from build123d import *

# Parameters (mm, degrees)
SKETCH_1_R          = 50
SKETCH_1_R_2        = 45
EXTRUDE_1_DEPTH     = 12
FILLET_1_R          = 80
CUT_EXTRUDE_1_DEPTH = 12
SKETCH_4_W          = 6
SKETCH_4_H          = 50
CUT_EXTRUDE_2_DEPTH = 12


with BuildPart() as part:
    # 草图1 → 凸台-拉伸1 (new body)
    with BuildSketch(Plane(origin=(0, 0, 0), x_dir=(0, 0, -1), z_dir=(1, 0, 0))):
        with BuildLine():
            Line((-150, 75), (560.88072706, 75))
            Line((560.88072706, 75), (948, -121.211138337))
            Line((948, -121.211138337), (1008, -163))
            Line((1008, -163), (1008, -168))
            Line((1008, -168), (998.615528128, -168))
            ThreePointArc((998.615528128, -168), (933.656897839, -200.339106398), (984, -252.598206242))
            Line((984, -252.598206242), (978, -260))
            Line((978, -260), (718, -260))
            Line((718, -260), (558, -175))
            Line((558, -175), (-150, -175))
            Line((-150, -175), (-150, 75))
        make_face()
        Circle(SKETCH_1_R, mode=Mode.SUBTRACT)
        with Locations((677, -50)):
            Circle(SKETCH_1_R_2, mode=Mode.SUBTRACT)
    extrude(amount=EXTRUDE_1_DEPTH)

    # 圆角1
    fillet_1_edges = [part.edges().sort_by_distance(p)[0] for p in [
        (6, -175, 150),
    ]]
    fillet(fillet_1_edges, radius=FILLET_1_R)

    # 草图3 → 切除-拉伸1 (cut)
    with BuildSketch(Plane(origin=(12, 0, 0), x_dir=(0, 0, -1), z_dir=(1, 0, 0))):
        with BuildLine():
            Line((-75, -92.5), (75, -92.5))
            ThreePointArc((75, -92.5), (82.5, -100), (75, -107.5))
            Line((75, -107.5), (-75, -107.5))
            ThreePointArc((-75, -107.5), (-82.5, -100), (-75, -92.5))
        make_face()
    extrude(amount=-CUT_EXTRUDE_1_DEPTH, mode=Mode.SUBTRACT)

    # 草图4 → 切除-拉伸2 (cut)
    with BuildSketch(Plane(origin=(12, 0, 0), x_dir=(0, 0, -1), z_dir=(1, 0, 0))):
        Polygon((170.51068381, 36.627050799), (206.580049862, 2.000459389), (202.424858893, -2.327864537), (166.355492841, 32.298726872), align=None)
        with Locations((297, 25)):
            Rectangle(SKETCH_4_W, SKETCH_4_H)
        Polygon((340.423834544, -33.569533818), (386.847669089, -52.139067635), (389.076013147, -46.56820749), (342.652178602, -27.998673672), align=None)
        Polygon((470.060094707, -91.936220159), (519.439680826, -99.788383854), (518.497421183, -105.713934188), (469.117835064, -97.861770494), align=None)
        Polygon((321.921336349, -68.379729076), (371.300922468, -76.231892771), (370.358662825, -82.157443105), (320.979076706, -74.305279411), align=None)
    extrude(amount=-CUT_EXTRUDE_2_DEPTH, mode=Mode.SUBTRACT)


solid = part.part
The listing builds one solid part. Answer for the finished solid, in the listing's coordinates (mm). A direction names the side the tool comes from. Give positions to 0.01 mm unless a question says otherwise; leave off trailing zeros. Order: outer loops, then holes, each group sorted by start corner. A loop starts at its lowest first (then second) coordinate and runs counter-clockwise, first axis right, second up. Notation, with made-up numbers: (84.5, -30.5) - (113.5, -30.5) arc R19 cw to (113.5, -4.5) - close; hole circle Ø2 at (-5, 80.25). An arc over 180 degrees is marked (long way). One line per item, written item: value. Start each with the question number.
1) A cutting plane is placed at C-C on x = 2. State how many separate pieces and enclosed holes the cut face has, then the cut area to 3 significant figures.
2) A cutting plane is placed at D-D on y = -235. Give the vertices of the cut face in (x, z), then the cut area to 3 significant figures.
3) A cutting plane is placed at A-A on z = -675. Give the vertices of the cut face in (x, y).
4) The mould has two halves that part along Z. Classify faces 1 (the face through (6.08, -150.94, 127.19)), 2 (the face through (6.084, -37.413, -366.189)), 3 (the face through (0, -90, -308)), 4 (the face through (5.916, -141.813, -977.58)): released by +Z, released by -Z, zero draft, split by the parting line, or undercut.
5) Given pin 1 Ø6 at (x, y) = (8, 30.5) entering from -Z; pin 2 Ø1.5 at (x, z) = (4.5, -171) entering from -Y; pin 3 Ø2 at (x, z) = (8.5, -716.5) entering from +Y, each flat-ended and moving along its own axis, determine where each tip first touches the part or whether it passes through.
6) A tool of negligible diameter and unlimited length cuts with its end or side. For faces 5 (the face through (5.916, -218.095, -639.12)), 6 (the face through (6.08, 19.56, -188.29)), from which of +Z, -Z, +X, -X, +Y, -Y can it reach the whole face along a straight path? Write none if from no direction.
7) A cutting plane is placed at B-B on z = -246. Give the vertices of the cut face in (x, y).
8) Find the intervals of material crossed by L1, parallel to Y at x = 9, z = 0; L2, parallel to Y at x = 9.5, z = 30; L3, parallel to Y at x = 11.5, z = -316, in increasing order.
Answer sheet:
1. separate pieces: 1
1. enclosed holes: 8
1. area: 244,000 mm2
2. outline: (0, -942) - (12, -942) - (12, -670.94) - (0, -670.94) - close
2. area: 3,250 mm2
3. outline: (0, -237.16) - (12, -237.16) - (12, -94.96) - (0, -94.96) - close; (0, -5.04) - (12, -5.04) - (12, 17.16) - (0, 17.16) - close
4. face 1: released by +Z
4. face 2: undercut
4. face 3: zero draft
4. face 4: released by -Z
5. pin 1: stops at z = -654.6
5. pin 2: stops at y = -175
5. pin 3: stops at y = -3.37
6. face 5: +Z, +X, -X, -Y
6. face 6: +X, -X
7. outline: (0, -175) - (12, -175) - (12, 75) - (0, 75) - close
8. L1: y = -175 to -107.5, -92.5 to -50, 50 to 75
8. L2: y = -175 to -107.5, -92.5 to -40, 40 to 75
8. L3: y = -175 to 75
